Geometry: final body of the model. Coordinates: model frame, mm. Coordinates: 2 decimals unless noted, no trailing zeros. Write each loop counter-clockwise with the first axis right and the second up, starting at its lowest first coordinate (ties: lowest second). Pieces come first, ordered by that corner, then holes. Notation, with made-up numbers: (35, 7) -> (81, 7) arc R15 cw to (81, 26) -> close; hole circle Ø3 at (76, 21.5). An arc over 180 degrees is marked (long way). One line per item, written item: value. Start each with the question number.
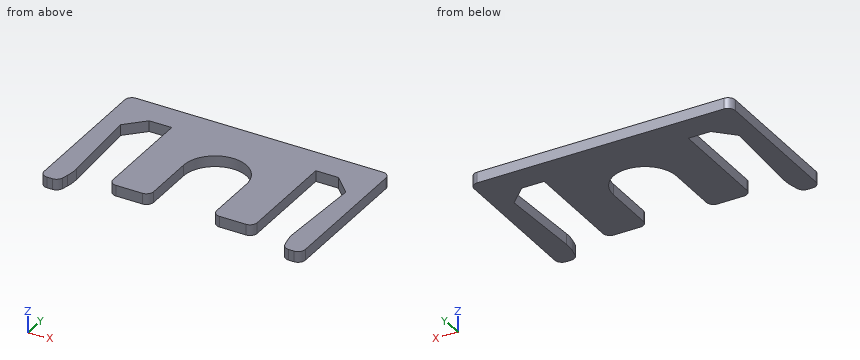
from build123d import *

# Parameters (mm, degrees)
BOSS_EXTRUDE1_DEPTH = 1.2
FILLET1_R           = 5
FILLET2_R           = 0.8


with BuildPart() as part:
    # Sketch1 → Boss-Extrude1 (new body)
    with BuildSketch(Plane.XY):
        with BuildLine():
            Line((-10.5, 0), (-12.5, -2))
            Line((-12.5, -2), (-12, -12))
            Line((-12, -12), (-12.5, -14))
            Line((-12.5, -14), (-14.5, -14))
            Line((-14.5, -14), (-14.5, 3))
            Line((-14.5, 3), (-12.5, 3))
            Line((-12.5, 3), (12.5, 3))
            Line((12.5, 3), (14.5, 3))
            Line((14.5, 3), (14.5, -14))
            Line((14.5, -14), (12.5, -14))
            Line((12.5, -14), (12, -12))
            Line((12, -12), (12.5, -2))
            Line((12.5, -2), (10.5, 0))
            Line((10.5, 0), (8, 0))
            Line((8, 0), (8, -12))
            Line((8, -12), (3.5, -12))
            Line((3.5, -12), (3.5, -5.5))
            ThreePointArc((3.5, -5.5), (0, -2), (-3.5, -5.5))
            Line((-3.5, -5.5), (-3.5, -12))
            Line((-3.5, -12), (-8, -12))
            Line((-8, -12), (-8, 0))
            Line((-8, 0), (-10.5, 0))
        make_face()
    extrude(amount=BOSS_EXTRUDE1_DEPTH)

    # Fillet1
    fillet1_edges = [part.edges().sort_by_distance(p)[0] for p in [
        (-12, -12, 0.6),
        (12, -12, 0.6),
    ]]
    fillet(fillet1_edges, radius=FILLET1_R)

    # Fillet2
    fillet2_edges = [part.edges().sort_by_distance(p)[0] for p in [
        (-12.5, -14, 0.6),
        (-14.5, -14, 0.6),
        (-14.5, 3, 0.6),
        (14.5, 3, 0.6),
        (14.5, -14, 0.6),
        (12.5, -14, 0.6),
        (8, -12, 0.6),
        (3.5, -12, 0.6),
        (-3.5, -12, 0.6),
        (-8, -12, 0.6),
    ]]
    fillet(fillet2_edges, radius=FILLET2_R)


solid = part.part
Q1. Cut plane A-A on y = -1.5. Output: boundary loops of the cut face in (x, z).
Q2. Cut plane D-D on x = -9.5. Output: boundary loops of the cut face in (y, z).
Q3. First-contact query: P1, Ø0.6, axis at x = -5.5, z = 0.5, coming from the -Y side; P2, Ø3, axis at x = -2.5, y = -8.5, coming from the +Z side. Flat tips, straight axial feed; report the tip coordinate or a pass-through.
Q4. Cut plane C-C on y = -6.5. Output: boundary loops of the cut face in (x, z) (3 decimals), and give its area (3 significant figures).
Q5. Line query: L1, parallel to X at y = -4, z = 0.45; L2, parallel to X at y = -3, z = 0.65; L3, parallel to X at y = -0.5, z = 0.6. Output: solid intervals per line, ascending. Write a range as from..to.
Solution:
1. outline: (-14.5, 0) -> (-12, 0) -> (-12, 1.2) -> (-14.5, 1.2) -> close; (-8, 0) -> (8, 0) -> (8, 1.2) -> (-8, 1.2) -> close; (12, 0) -> (14.5, 0) -> (14.5, 1.2) -> (12, 1.2) -> close
2. outline: (0, 0) -> (3, 0) -> (3, 1.2) -> (0, 1.2) -> close
3. P1: y = -12
3. P2: z = 1.2
4. outline: (-14.5, 0) -> (-12.275, 0) -> (-12.275, 1.2) -> (-14.5, 1.2) -> close; (-8, 0) -> (-3.5, 0) -> (-3.5, 1.2) -> (-8, 1.2) -> close; (3.5, 0) -> (8, 0) -> (8, 1.2) -> (3.5, 1.2) -> close; (12.275, 0) -> (14.5, 0) -> (14.5, 1.2) -> (12.275, 1.2) -> close
4. area: 16.1 mm²
5. L1: -14.5..-12.4, -8..-3.16, 3.16..8, 12.4..14.5
5. L2: -14.5..-12.45, -8..-2.45, 2.45..8, 12.45..14.5
5. L3: -14.5..-11, -8..8, 11..14.5
